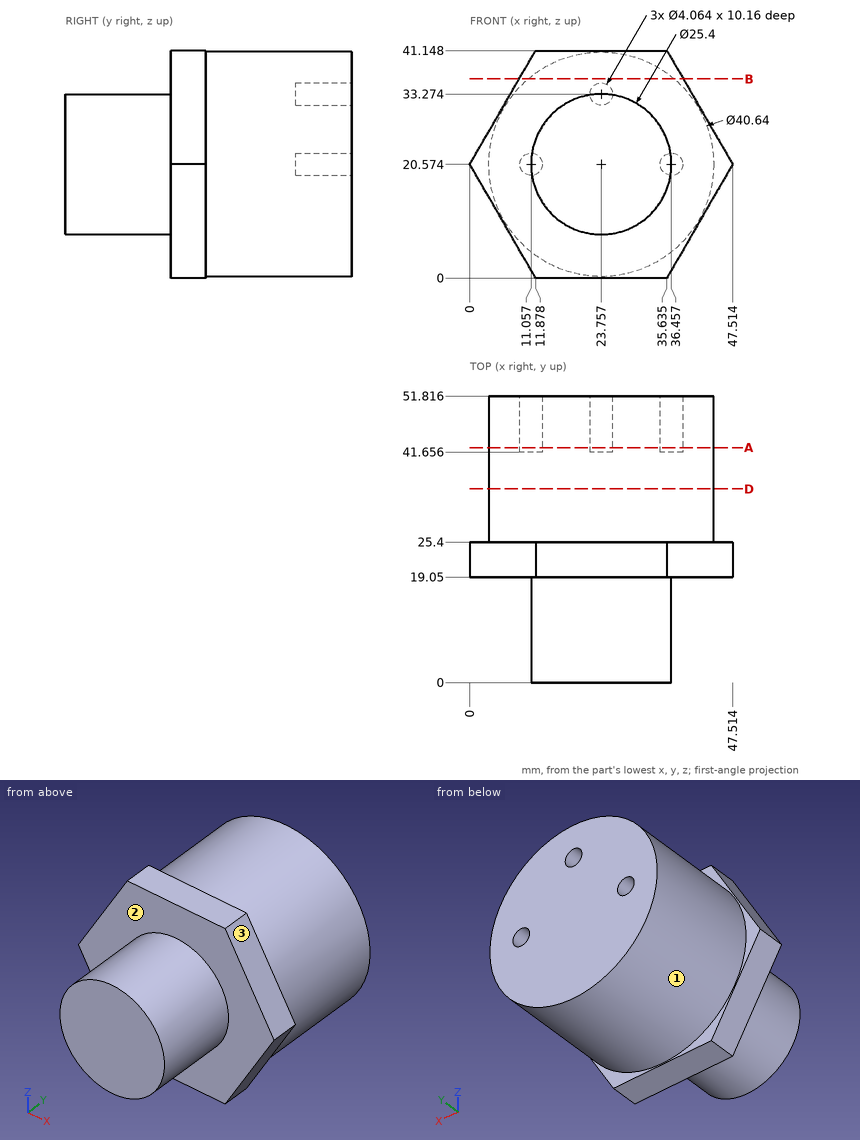
Design review of the part shown in the three views and the two pictorial views. Dimensions are in mm from the part's minimum x, y and z. A direction names the side the tool comes from. Round coordinates to 2 decimals unless told otherwise and drop trailing zeros. Order: outer loops, then holes, each group sorted by start corner. A loop starts at its lowest first (then second) coordinate and runs counter-clockwise, first axis right, second up.
(1) Take a section at A-A, the plane y = 42.5. State the section outline as (x, z) points, plus the area to 3 significant figures.
Working result:
outline: circle Ø40.64 at (23.76, 20.57); hole circle Ø4.06 at (11.06, 20.57); hole circle Ø4.06 at (23.76, 33.27); hole circle Ø4.06 at (36.46, 20.57)
area: 1,260 mm2
(2) For P1, Ø8, axis at x = 26, y = 35, coming from the +Z side; P2, Ø6, axis at y = 8.5, z = 4, coming from the -X side; P3, Ø2.5, axis at x = 11.06, z = 20.57, coming from the +Y side; P4, Ø3, axis at x = 10, y = 34.5, coming from the +Z side, all flat-tipped, find the tip position at first contact; note any pin that passes through.
Working result:
P1: stops at z = 40.89
P2: passes through
P3: stops at y = 41.66
P4: stops at z = 36.78
(3) Take a section at D-D, the plane y = 35. State the section outline as (x, z) points, plus the area to 3 significant figures.
Working result:
outline: circle Ø40.64 at (23.76, 20.57)
area: 1,300 mm2
(4) Take a section at B-B, the plane z = 36. State the section outline as (x, y) points, plus the area to 3 significant figures.
Working result:
outline: (8.91, 19.05) - (38.61, 19.05) - (38.61, 25.4) - (36.98, 25.4) - (36.98, 51.82) - (10.53, 51.82) - (10.53, 25.4) - (8.91, 25.4) - close
area: 887 mm2
(5) Tool access review of the marked faces 1, 2 and 3: name each direction out of +Z, -Z, +X, -X, +Y, -Y from which nothing blocks a thin tool from reaching the whole face with its end or side.
Working result:
face 1: +Y
face 2: -Y
face 3: +Z, +X, +Y, -Y
(6) Wall thickness on L1, parallel to Y at x = 37, z = 26; L2, parallel to Y at x = 45.5, z = 22.5; L3, parallel to Z at x = 40.5, y = 41 (1 decimal): over which ranges is each line inside the solid? List them lowest first.
Working result:
L1: y = 19.05 to 51.82
L2: y = 19.05 to 25.4
L3: z = 9.1 to 32.1
